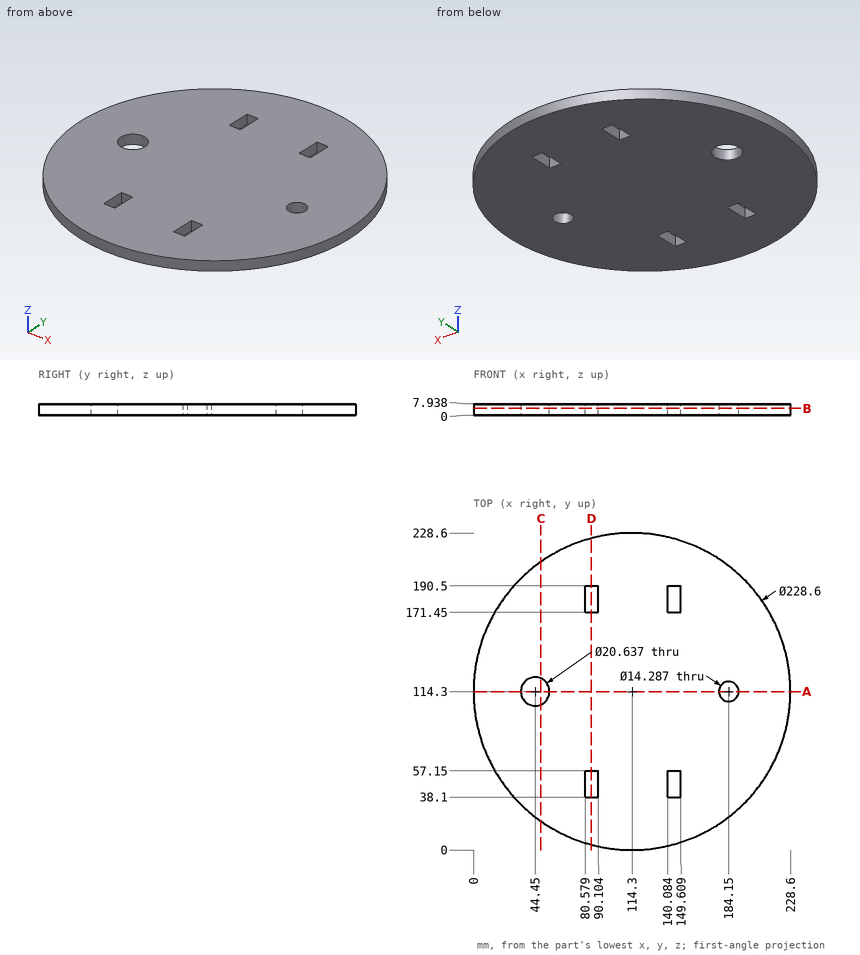
Study the drawing (mm; zero at the part's minimum x, y, z) and answer. Coordinates: 2 decimals unless noted, no trailing zeros. Write each loop counter-clockwise with the first axis right and the second up, starting at its lowest first coordinate (ties: lowest second). Pieces come first, ordered by that corner, then holes. Notation, with made-up numbers: M 59.25,-15.75 L 91.25,-15.75 A26 ccw 91.25,11.25 Z; hole C -22.5,86.25 d2. An arc over 180 degrees is marked long. Use one line per item in the form item = value.
Item 1: Find section A-A, the plane y = 114.3. Give the vertices of the cut face in (x, z), plus the area to 3 significant figures.
Model answer:
outline = M 0,0 L 34.13,0 L 34.13,7.94 L 0,7.94 Z; M 54.77,0 L 177.01,0 L 177.01,7.94 L 54.77,7.94 Z; M 191.29,0 L 228.6,0 L 228.6,7.94 L 191.29,7.94 Z
area = 1,540 mm2
Item 2: Given P1, Ø2.5, axis at x = 146.5, z = 3.5, coming from the +Y side; P2, Ø4, axis at y = 53.5, z = 6.5, coming from the +X side (1 decimal); P3, Ø1.5, axis at x = 135, z = 6, coming from the +Y side (1 decimal); P4, Ø1.5, axis at x = 199.5, y = 35.5, coming from the -Z side, each flat-ended and moving along its own axis, determine where each tip first touches the part or whether it passes through.
Model answer:
P1 = 224.33
P2 = 212.3
P3 = 226.8
P4 = through
Item 3: Find section B-B, the plane z = 4.75. Give the vertices of the cut face in (x, y), plus the area to 3 significant figures.
Model answer:
outline = C 114.3,114.3 d228.6; hole C 44.45,114.3 d20.64; hole M 80.58,38.1 L 90.1,38.1 L 90.1,57.15 L 80.58,57.15 Z; hole M 80.58,171.45 L 90.1,171.45 L 90.1,190.5 L 80.58,190.5 Z; hole M 140.08,38.1 L 149.61,38.1 L 149.61,57.15 L 140.08,57.15 Z; hole M 140.08,171.45 L 149.61,171.45 L 149.61,190.5 L 140.08,190.5 Z; hole C 184.15,114.3 d14.29
area = 39,800 mm2
Item 4: Find the intervals of material crossed by probe 1 along X at (y, z) = (51.5, 7.25) (1 decimal); probe 2 along X at (y, z) = (50.5, 6.5) (1 decimal); probe 3 along Y at (x, z) = (184.15, 4) (1 decimal), in increasing order.
Model answer:
probe_1 = 18.8 to 80.6, 90.1 to 140.1, 149.6 to 209.8
probe_2 = 19.5 to 80.6, 90.1 to 140.1, 149.6 to 209.1
probe_3 = 23.8 to 107.2, 121.4 to 204.8
Item 5: Find section D-D, the plane x = 85. Give the vertices of the cut face in (y, z), plus the area to 3 significant figures.
Model answer:
outline = M 3.82,0 L 38.1,0 L 38.1,7.94 L 3.82,7.94 Z; M 57.15,0 L 171.45,0 L 171.45,7.94 L 57.15,7.94 Z; M 190.5,0 L 224.78,0 L 224.78,7.94 L 190.5,7.94 Z
area = 1,450 mm2
Item 6: Find section C-C, the plane x = 48.5. Give the vertices of the cut face in (y, z).
Model answer:
outline = M 20.84,0 L 104.81,0 L 104.81,7.94 L 20.84,7.94 Z; M 123.79,0 L 207.76,0 L 207.76,7.94 L 123.79,7.94 Z
